from build123d import *

# Parameters (mm, degrees)
EXTRUDE_2_DEPTH     = 3
CUT_EXTRUDE_1_DEPTH = 3
CUT_EXTRUDE_2_DEPTH = 3
CUT_EXTRUDE_3_DEPTH = 1
SKETCH_16_R         = 85.646074049
CUT_EXTRUDE_6_DEPTH = 10
EXTRUDE_3_DEPTH     = 20
FILLET_1_R          = 5
SKETCH_14_R         = 1.25
SKETCH_14_W         = 3
SKETCH_14_H         = 15
CUT_EXTRUDE_8_DEPTH = 10
CUT_EXTRUDE_9_DEPTH = 10
FILLET_2_R          = 1


with BuildPart() as part:
    # 草图4 → 凸台-拉伸2 (new body)
    with BuildSketch(Plane(origin=(0, 0, 0), x_dir=(1, 0, 0), z_dir=(0, 1, 0))):
        with BuildLine():
            Line((0, 0), (135, 0))
            ThreePointArc((135, 0), (95.45941546, -95.45941546), (0, -135))
            Line((0, -135), (0, 0))
        make_face()
    extrude(amount=EXTRUDE_2_DEPTH)

    # 草图6 → 切除-拉伸1 (cut)
    with BuildSketch(Plane(origin=(0, 3, 0), x_dir=(1, 0, 0), z_dir=(0, 1, 0))):
        with BuildLine():
            Line((0, 0), (85, 0))
            ThreePointArc((85, 0), (69.910657271, -48.347699015), (30, -79.529868603))
            Line((30, -79.529868603), (47.647058824, -126.312144252))
            ThreePointArc((47.647058824, -126.312144252), (24.216322244, -132.810277227), (0, -135))
            Line((0, -135), (0, -18))
            Line((0, -18), (0, 0))
        make_face()
    extrude(amount=-CUT_EXTRUDE_1_DEPTH, mode=Mode.SUBTRACT)

    # 草图8 → 切除-拉伸2 (cut)
    with BuildSketch(Plane(origin=(0, 3, 0), x_dir=(1, 0, 0), z_dir=(0, 1, 0))):
        with BuildLine():
            Line((45.882352941, -121.633916687), (76.908655449, -110.950703995))
            ThreePointArc((76.908655449, -110.950703995), (62.749700806, -119.530226507), (47.647058824, -126.312144252))
            Line((47.647058824, -126.312144252), (45.882352941, -121.633916687))
        make_face()
    extrude(amount=-CUT_EXTRUDE_2_DEPTH, mode=Mode.SUBTRACT)

    # 草图9 → 切除-拉伸3 (cut)
    with BuildSketch(Plane(origin=(0, 3, 0), x_dir=(1, 0, 0), z_dir=(0, 1, 0))):
        with BuildLine():
            Line((40.588235294, -107.599233992), (30, -79.529868603))
            ThreePointArc((30, -79.529868603), (69.910657271, -48.347699015), (85, 0))
            Line((85, 0), (115, 0))
            ThreePointArc((115, 0), (96.045984502, -66.421952411), (40.588235294, -107.599233992))
        make_face()
    extrude(amount=-CUT_EXTRUDE_3_DEPTH, mode=Mode.SUBTRACT)

    # 草图16 → 切除-拉伸6 (cut)
    with BuildSketch(Plane(origin=(0, 2, 0), x_dir=(1, 0, 0), z_dir=(0, 1, 0))):
        with Locations((0, -10.5)):
            Circle(SKETCH_16_R)
    extrude(amount=-CUT_EXTRUDE_6_DEPTH, mode=Mode.SUBTRACT)

    # 草图13 → 凸台-拉伸3 (add)
    with BuildSketch(Plane(origin=(0, 0, 0), x_dir=(-1, 0, 0), z_dir=(0, 0, -1))):
        Polygon((-135, 3), (-135, 0), (-85, 0), (-85, 2), (-115, 2), (-115, 3), align=None)
    extrude(amount=EXTRUDE_3_DEPTH)

    # 圆角1
    fillet_1_edges = [part.edges().sort_by_distance(p)[0] for p in [
        (45.882352941, 1.5, 121.633916687),
        (135, 1.5, -20),
    ]]
    fillet(fillet_1_edges, radius=FILLET_1_R)

    # 草图14 → 切除-拉伸8 (cut)
    with BuildSketch(Plane(origin=(0, 3, 0), x_dir=(1, 0, 0), z_dir=(0, 1, 0))):
        with Locations((129.5, -17)):
            Circle(SKETCH_14_R)
        with Locations((129.5, -8)):
            Circle(SKETCH_14_R)
        with Locations((56.761619346, -113.641470943)):
            Circle(SKETCH_14_R)
        with Locations((65.182428963, -110.465000355)):
            Circle(SKETCH_14_R)
        with Locations((118, -12.5)):
            Rectangle(SKETCH_14_W, SKETCH_14_H)
        Polygon((50.425271043, -105.343839343), (49.366447513, -102.536902804), (63.401130208, -97.242785157), (64.459953737, -100.049721696), align=None)
    extrude(amount=-CUT_EXTRUDE_8_DEPTH, mode=Mode.SUBTRACT)

    # 草图17 → 切除-拉伸9 (cut)
    with BuildSketch(Plane(origin=(0, 3, 0), x_dir=(1, 0, 0), z_dir=(0, 1, 0))):
        with BuildLine():
            Line((115.911099155, -31.058285412), (125.570357418, -33.646475863))
            ThreePointArc((125.570357418, -33.646475863), (119.21780967, -51.83737896), (110.2462525, -68.88950435))
            Line((110.2462525, -68.88950435), (101.765771539, -63.590311708))
            ThreePointArc((101.765771539, -63.590311708), (110.047208926, -47.849888271), (115.911099155, -31.058285412))
        make_face()
        with BuildLine():
            Line((73.879377039, -94.561290433), (80.035991792, -102.441397969))
            ThreePointArc((80.035991792, -102.441397969), (94.298668232, -89.48609484), (106.489765758, -74.564936726))
            Line((106.489765758, -74.564936726), (98.298245315, -68.829172362))
            ThreePointArc((98.298245315, -68.829172362), (87.044924521, -82.602549083), (73.879377039, -94.561290433))
        make_face()
    extrude(amount=-CUT_EXTRUDE_9_DEPTH, mode=Mode.SUBTRACT)

    # 圆角2
    fillet_2_edges = [part.edges().sort_by_distance(p)[0] for p in [
        (73.879377039, 1.5, 94.561290433),
        (98.298245315, 1.5, 68.829172362),
        (106.489765758, 1.5, 74.564936726),
        (80.035991792, 1.5, 102.441397969),
        (101.765771539, 1.5, 63.590311708),
        (115.911099155, 1.5, 31.058285412),
        (125.570357418, 1.5, 33.646475863),
        (110.2462525, 1.5, 68.88950435),
    ]]
    fillet(fillet_2_edges, radius=FILLET_2_R)


solid = part.part
Input: part model. Units: mm. Frame: model coordinates. A direction names the side the tool comes from. Coordinates: 2 decimals unless noted, no trailing zeros. Order: outer loops, then holes, each group sorted by start corner. A loop starts at its lowest first (then second) coordinate and runs counter-clockwise, first axis right, second up. Notation, with made-up numbers: M -6.75,27 L 21.25,27 A23 ccw 21.25,60 Z; hole C -35.75,70.25 d5. An arc over 180 degrees is marked long. Answer in a Markdown table with one row per item.
(1) Section query C-C, the plane x = 60.5. Output: boundary loops of the cut face in (y, z), plus the area to 3 significant figures.
Numbers:
| item | result |
|---|---|
| outline | M 0,71.12 L 2,71.12 L 2,98.34 L 0,98.34 Z; M 0,101.54 L 3,101.54 L 3,116.6 L 0,116.6 Z |
| area | 99.6 mm^2 |
(2) Contact query for flat-ended pins moving along their axis: pin 1 Ø1 at (y, z) = (1, -13) entering from -X; pin 2 Ø1.5 at (x, z) = (129.5, 17) entering from +Y; pin 3 Ø1 at (x, y) = (83.5, 1) entering from +Z; pin 4 Ø1.5 at (x, y) = (71.5, 2) entering from +Z. Output: stop coordinate, or through.
Numbers:
| item | result |
|---|---|
| pin 1 | stops at x = 85 |
| pin 2 | passes through |
| pin 3 | stops at z = 106.47 |
| pin 4 | stops at z = 113.07 |
(3) Draft query along Z for faces 4 (the flat face through (120.683, 1.521, 32.337)), 5 (the flat face through (135, 2, -7)), 6 (the flat face through (38.844, 1.188, 102.976)). Return one class per face: pulls with the +Z half, pulls with the -Z half, needs draft (parallel to the pull), parting line crosses it, or undercut.
Numbers:
| item | result |
|---|---|
| face 4 | undercut |
| face 5 | needs draft |
| face 6 | pulls with the +Z half |
(4) Material intervals for line 1 (X direction, y = 1.85, z = 8); line 2 (X direction, y = 1.85, z = 17); line 3 (Z direction, x = 102.5, y = 0.6), sorted ascending. Write a range as [from, to].
Numbers:
| item | result |
|---|---|
| line 1 | x = [85.61, 116.5], [119.5, 128.25], [130.75, 134.76] |
| line 2 | x = [85.4, 116.5], [119.5, 128.25], [130.75, 133.93] |
| line 3 | z = [-20, 62.4], [64.04, 71.77], [79.96, 87.86] |
(5) Section query A-A, the plane z = -10.5. Output: boundary loops of the cut face in (x, y).
Numbers:
| item | result |
|---|---|
| outline | M 85,0 L 135,0 L 135,3 L 115,3 L 115,2 L 85,2 Z |
(6) Section query D-D, the plane y = 1.4. Give the number of separate pieces and of enclosed holes in the cut face, plus the area to 3 significant figures.
Numbers:
| item | result |
|---|---|
| separate pieces | 1 |
| enclosed holes | 8 |
| area | 6,060 mm^2 |
(7) Section query B-B, the plane z = 51.5. Output: boundary loops of the cut face in (x, y).
Numbers:
| item | result |
|---|---|
| outline | M 75.19,0 L 108.39,0 L 108.39,3 L 104.68,3 L 104.68,2 L 75.19,2 Z; M 119.36,0 L 124.79,0 L 124.79,3 L 119.36,3 Z |
(8) Access query for faces 1 (the cylindrical face through (73.854, 1.014, 53.869)), 2 (the flat face through (119.5, 2, 13)), 3 (the flat face through (86, 2, 44)). Directions: +Z, -Z, +X, -X, +Y, -Y. A direction counts if a zero-diameter tool reaches every point of the face in a straight line with its end or side. Return the directions, or none.
Numbers:
| item | result |
|---|---|
| face 1 | -X, +Y, -Y |
| face 2 | +Y, -Y |
| face 3 | -Z, -X, +Y |
